```python
from build123d import *

# Parameters (mm, degrees)
BOSS_EXTRUDE1_DEPTH         = 2.54
BOSS_EXTRUDE1_DEPTH_BACK    = 1.27
SKETCH1_R                   = 3.96875
SKETCH1_R_2                 = 1.8288
SKETCH1_W                   = 41.843046883
SKETCH1_H                   = 42.037
SKETCH2_W                   = 41.843046883
SKETCH2_H                   = 1.3462
SKETCH2_H_2                 = 1.27
CUT_EXTRUDE1_DEPTH          = 239.72059927
F_43_0_089_DIAMETER_HOLE1_D = 2.2606


with BuildPart() as part:
    # Sketch1 → Boss-Extrude1 (new, two sides: drawn at the far end of the back side and taken through both)
    with BuildSketch(Plane(origin=(0, 0, 0), x_dir=(1, 0, 0), z_dir=(0, 1, 0)).offset(-BOSS_EXTRUDE1_DEPTH_BACK)):
        Polygon((0, -9.930453132), (0, 126.604027306), (116.61929014, 208.261733362), (116.61929014, 88.059530464), align=None)
        with Locations(Location((98.042383887, 108.299920281, 0), (0, 0, 270))):
            Circle(SKETCH1_R, mode=Mode.SUBTRACT)
        with Locations(Location((89.458607167, 133.716920501, 0), (0, 0, 270))):
            Circle(SKETCH1_R_2, mode=Mode.SUBTRACT)
        with Locations(Location((103.545290714, 133.716920501, 0), (0, 0, 270))):
            Circle(SKETCH1_R_2, mode=Mode.SUBTRACT)
        with Locations((63.903769784, 117.780411398)):
            Rectangle(SKETCH1_W, SKETCH1_H, mode=Mode.SUBTRACT)
    extrude(amount=BOSS_EXTRUDE1_DEPTH + BOSS_EXTRUDE1_DEPTH_BACK)

    # Sketch2 → Cut-Extrude1 (cut, through all)
    with BuildSketch(Plane(origin=(0, 2.54, 0), x_dir=(1, 0, 0), z_dir=(0, 1, 0))):
        with Locations((63.903769784, 96.088811398)):
            Rectangle(SKETCH2_W, SKETCH2_H)
        with Locations((63.903769784, 139.433911398)):
            Rectangle(SKETCH2_W, SKETCH2_H_2)
    extrude(amount=-CUT_EXTRUDE1_DEPTH, mode=Mode.SUBTRACT)

    # #43 (0.089) Diameter Hole1 (through all)
    with Locations(Plane(origin=(0, 2.54, 0), x_dir=(1, 0, 0), z_dir=(0, 1, 0))):
        with Locations((84.317293225, 95.923711398), (84.317293225, 139.560911398), (43.490246342, 95.923711398), (43.490246342, 139.560911398)):
            Hole(F_43_0_089_DIAMETER_HOLE1_D / 2)


solid = part.part
```
For this review, take the finished solid that the model builds, in its own axes (mm). A direction names the side the tool comes from. Give positions to 0.01 mm unless a question says otherwise; leave off trailing zeros. Write each loop counter-clockwise with the first axis right and the second up, starting at its lowest first coordinate (ties: lowest second). Pieces come first, ordered by that corner, then holes.
Item 1: Take a section at B-B (z = -129). Give the boundary of the cut face in (x, y), and give its area (3 significant figures).
Item 2: Wall thickness on probe 1 along X at (y, z) = (0.35, -121.5); probe 2 along Z at (x, y) = (54.5, 2.25); probe 3 along Z at (x, y) = (65, 0.65): over which ranges is each line inside the solid? List them lowest first.
Item 3: Take a section at A-A (x = 54). Give the boundary of the cut face in (y, z).
Item 4: The part is to be moulded in two halves that separate along X. For faces 3 (the face through (0, 1, -57)), 4 (the face through (64, 1, -95.416)), 5 (the face through (42.982, 1, -117)), 6 (the face through (33, 2.54, -101)), say which applies: +X half, -X half, draft (parallel to the pull), parting line (faces both ways), or undercut.
Item 5: Machinability: for faces 1 (the face through (84.825, 1, -117)), 2 (the face through (33, -1.27, -101)), which of the approach directions +Z, -Z, +X, -X, +Y, -Y give a long, thin tool a straight path to every point of the face, cutting with its end or side? Answer none if there is none.
Item 6: Take a section at C-C (y = -0.2). Give the boundary of the cut face in (x, z), and give its area (3 significant figures).
Item 7: Take a section at D-D (z = -31.5). Give the boundary of the cut face in (x, y), and give its area (3 significant figures).
Item 8: Insertion check: P1, Ø2.5, axis at x = 43.49, z = -95.92, coming from the +Y side; P2, Ø1.4, axis at x = 43.49, z = -139.56, coming from the -Y side; P3, Ø1.9, axis at x = 67, y = 0.5, coming from the -Z side. Each pin has a flat end and moves straight along its axis. Give the tip position at first contact, or say it passes through.
Established:
1. outline: (3.42, -1.27) - (42.98, -1.27) - (42.98, 2.54) - (3.42, 2.54) - close; (84.83, -1.27) - (116.62, -1.27) - (116.62, 2.54) - (84.83, 2.54) - close
1. area: 272 mm2
2. probe 1: x = 0 to 42.98, 84.83 to 116.62
2. probe 2: z = -164.77 to -140.07, -95.42 to -35.86
2. probe 3: z = -172.12 to -140.07, -95.42 to -44.69
3. outline: (-1.27, -164.42) - (2.54, -164.42) - (2.54, -140.07) - (-1.27, -140.07) - close; (-1.27, -95.42) - (2.54, -95.42) - (2.54, -35.44) - (-1.27, -35.44) - close
4. face 3: -X half
4. face 4: undercut
4. face 5: undercut
4. face 6: draft
5. face 1: +Y, -Y
5. face 2: +Z, -Z, +X, -X, -Y
6. outline: (0, -126.6) - (116.62, -208.26) - (116.62, -88.06) - (0, 9.93) - close; hole (42.98, -138.55) arc R1.13 ccw (long way) to (44.5, -140.07) - (83.31, -140.07) arc R1.13 ccw (long way) to (84.83, -138.55) - (84.83, -96.93) arc R1.13 ccw (long way) to (83.31, -95.42) - (44.5, -95.42) arc R1.13 ccw (long way) to (42.98, -96.93) - close; hole circle Ø3.66 at (89.46, -133.72); hole circle Ø7.94 at (98.04, -108.3); hole circle Ø3.66 at (103.55, -133.72)
6. area: 13,000 mm2
7. outline: (0, -1.27) - (49.31, -1.27) - (49.31, 2.54) - (0, 2.54) - close
7. area: 188 mm2
8. P1: stops at y = 2.54
8. P2: passes through
8. P3: stops at z = -174.18
